For this review, take the finished solid that the model builds, in its own axes (mm). Give positions to 0.01 mm unless a question says otherwise; leave off trailing zeros. Order: outer loops, then holes, each group sorted by start corner. A loop starts at its lowest first (then second) coordinate and runs counter-clockwise, first axis right, second up. Notation, with made-up numbers: M 28.25,-38 L 54.25,-38 A27 ccw 54.25,-15 Z; hole C 14.25,77.25 d8. An arc over 180 degrees is marked long. Answer as CSV lines item,"result". Start each with the question number.
1. We need section A-A, the plane y = -6.75. Give the boundary of the cut face in (x, z).
2. We need section B-B, the plane x = 3.81. Give the boundary of the cut face in (y, z), and give its area (4 significant figures).
3. We need section D-D, the plane x = 5. Give the boundary of the cut face in (y, z).
4. For line 1 along Z through (x, y) = (3, -8.25); line 2 along X through (y, z) = (-4.75, 3); line 3 along X through (y, z) = (-1, 2.75), list the stretches that pass through material, from the lowest coordinate up.
5. We need section C-C, the plane z = 2.5. State how many separate pieces and enclosed holes the cut face has, and give its area (3 significant figures).
6. Clearance check with flat-ended pins moving along their axes: P1, Ø4, axis at x = 5, y = -12.5, coming from the -Z side; P2, Ø0.6, axis at x = 0.5, z = -1.5, coming from the -Y side; P3, Ø1, axis at y = -13, z = 4, coming from the +X side; P4, Ø1.1, axis at y = 1.5, z = 7, coming from the -X side. State where each tip first meets the part, or that it passes through.
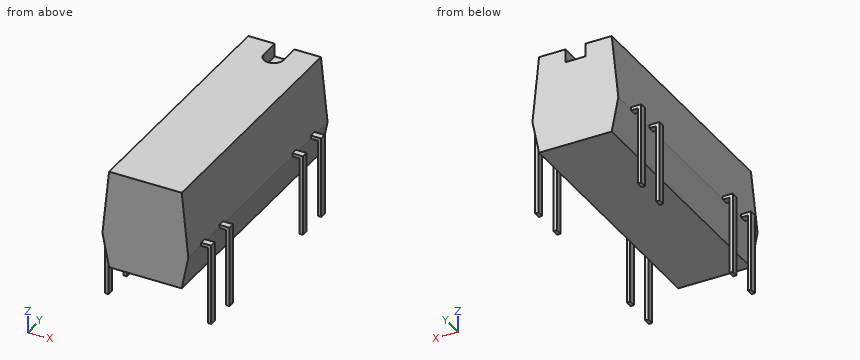
from build123d import *

# Parameters (mm, degrees)
PAD003_DEPTH = 0.25
PAD_DEPTH    = 9.65
POCKET_DEPTH = 1
PAD002_DEPTH = 0.25
PAD001_DEPTH = 0.25
PAD004_DEPTH = 0.25


with BuildPart() as pad003:
    # Sketch004 → Pad003 (new body, symmetric)
    with BuildSketch(Plane.XZ.offset(2.54)):
        Polygon((-0.2, -3.2), (0.05, -3.2), (0.05, 2.7), (7.57, 2.7), (7.57, -3.2), (7.82, -3.2), (7.82, 2.95), (-0.2, 2.95), align=None)
    extrude(amount=PAD003_DEPTH, both=True)


with BuildPart() as pocket:
    # Sketch → Pad (new body, symmetric)
    with BuildSketch(Plane.XZ.offset(7.62)):
        Polygon((1.06, 0.2), (6.56, 0.2), (7.06, 2.75), (6.56, 7.7), (1.06, 7.7), (0.56, 2.75), align=None)
    extrude(amount=PAD_DEPTH, both=True)

    # Sketch003 → Pocket (cut)
    with BuildSketch(Plane(origin=(0, -7.62, 7.7), x_dir=(-1, 0, 0), z_dir=(0, 0, 1))):
        with BuildLine():
            ThreePointArc((-3.06, -8.15), (-3.81, -7.4), (-4.56, -8.15))
            Line((-4.56, -8.15), (-4.56, -9.65))
            Line((-4.56, -9.65), (-3.06, -9.65))
            Line((-3.06, -9.65), (-3.06, -8.15))
        make_face()
    extrude(amount=-POCKET_DEPTH, mode=Mode.SUBTRACT)


with BuildPart() as pad002:
    # Sketch002 → Pad002 (new body, symmetric)
    with BuildSketch(Plane.XZ.offset(15.24)):
        Polygon((-0.2, -3.2), (0.05, -3.2), (0.05, 2.7), (7.57, 2.7), (7.57, -3.2), (7.82, -3.2), (7.82, 2.95), (-0.2, 2.95), align=None)
    extrude(amount=PAD002_DEPTH, both=True)


with BuildPart() as pad001:
    # Sketch001 → Pad001 (new body, symmetric)
    with BuildSketch(Plane.XZ):
        Polygon((-0.2, -3.2), (0.05, -3.2), (0.05, 2.7), (7.57, 2.7), (7.57, -3.2), (7.82, -3.2), (7.82, 2.95), (-0.2, 2.95), align=None)
    extrude(amount=PAD001_DEPTH, both=True)


with BuildPart() as obj1:
    # Sketch005 → Pad004 (new body, symmetric)
    with BuildSketch(Plane.XZ.offset(12.7)):
        Polygon((-0.2, -3.2), (0.05, -3.2), (0.05, 2.7), (7.57, 2.7), (7.57, -3.2), (7.82, -3.2), (7.82, 2.95), (-0.2, 2.95), align=None)
    extrude(amount=PAD004_DEPTH, both=True)

    add(pad003.part)
    add(pocket.part)
    add(pad002.part)
    add(pad001.part)


solid = obj1.part
Result set:
1,outline,"M 0.56,2.75 L 1.06,0.2 L 6.56,0.2 L 7.06,2.75 L 6.56,7.7 L 1.06,7.7 Z"
2,outline,"M -17.27,0.2 L 2.03,0.2 L 2.03,6.7 L -0.22,6.7 L -0.22,7.7 L -17.27,7.7 Z"
2,area,"142.5 mm2"
3,outline,"M -17.27,0.2 L 2.03,0.2 L 2.03,7.7 L -17.27,7.7 Z"
4,line 1,"0.2 to 7.7"
4,line 2,"0.59 to 7.03"
4,line 3,"0.56 to 7.06"
5,separate pieces,"9"
5,enclosed holes,"0"
5,area,"125 mm2"
6,P1,"z = 0.2"
6,P2,"through"
6,P3,"x = 6.98"
6,P4,"x = 0.93"
